For this review, take the finished solid that the model builds, in its own axes (mm). A direction names the side the tool comes from. Coordinates: 2 decimals unless noted, no trailing zeros. Loops run counter-clockwise (first coordinate to the right, second up) from the corner with the lowest first, then second, coordinate; pieces in that order, holes last.
1. Take a section at B-B, the plane y = -2. State the section outline as (x, z) points, then the cut area to 3 significant figures.
2. To check wall thickness, follow probe 1 along Y at (x, z) = (0, 42); probe 2 along Z at (x, y) = (10, 0); probe 3 along Y at (x, z) = (-9, 43.5). State the ranges of each line that lie inside material, in increasing order.
3. Clearance check with flat-ended pins moving along their axes: P1, Ø2.5, axis at y = -9.5, z = 8, coming from the +X side; P2, Ø8, axis at x = -5, z = 22, coming from the +Y side; P3, Ø8, axis at y = 5, z = 23, coming from the +X side; P4, Ø4, axis at x = 6, y = 24.5, coming from the -Z side. State where each tip first meets the part, or that it passes through.
4. Take a section at A-A, the plane x = -3.5. State the section outline as (y, z) points.
5. Take a section at D-D, the plane y = 23.5. State the section outline as (x, z) points, then the cut area to 3 significant figures.
6. Mouldability with a two-part tool opening along Y and no side actions: class faces 1 (the face through (-10.319, -9, 25)), 2 (the face through (0, -11, 6.35)), 3 (the face through (9, -10.319, 25)) as pulls with the +Y half, pulls with the -Y half, needs draft (parallel to the pull), parting line crosses it, or undercut.
7. Machinability: for faces 4 (the face through (0.593, 24.74, 3.188)), 5 (the face through (-9.79, 8.96, 7.67)), 6 (the face through (-0.1, -12.7, 10.4)), which of the approach directions +Z, -Z, +X, -X, +Y, -Y give a long, thin tool a straight path to every point of the face, cutting with its end or side? Answer none if there is none.
8. Take a section at C-C, the plane z = 35. State the section outline as (x, y) points.
```python
from build123d import *

# Parameters (mm, degrees)
SKETCH1_R               = 16.66875
BOSS_EXTRUDE1_DEPTH     = 50.8
SKETCH2_R               = 16.66875
BOSS_EXTRUDE2_DEPTH     = 34.13125
SKETCH3_R               = 16.66875
BOSS_EXTRUDE3_DEPTH     = 34.13125
CUT_EXTRUDE1_DEPTH      = 71.075134343
CUT_EXTRUDE1_DEPTH_BACK = 71.075134343
CUT_EXTRUDE2_DEPTH      = 80.537552304
SKETCH8_R               = 12.7
CUT_EXTRUDE3_DEPTH      = 44.45
SKETCH9_R               = 13.49375
CUT_EXTRUDE4_DEPTH      = 19.05
SKETCH10_R              = 12.7
CUT_EXTRUDE5_DEPTH      = 44.45
SKETCH11_R              = 13.49375
CUT_EXTRUDE6_DEPTH      = 19.05
SKETCH12_R              = 12.7
CUT_EXTRUDE7_DEPTH      = 44.45
SKETCH13_R              = 13.49375
CUT_EXTRUDE8_DEPTH      = 19.05


with BuildPart() as part:
    # Sketch1 → Boss-Extrude1 (new body)
    with BuildSketch(Plane.XY):
        Circle(SKETCH1_R)
    extrude(amount=BOSS_EXTRUDE1_DEPTH)

    # Sketch2 → Boss-Extrude2 (add)
    with BuildSketch(Plane(origin=(0, 0, 0), x_dir=(0, 0, -1), z_dir=(1, 0, 0))):
        with Locations((-16.66875, 0)):
            Circle(SKETCH2_R)
    extrude(amount=BOSS_EXTRUDE2_DEPTH)

    # Sketch3 → Boss-Extrude3 (add)
    with BuildSketch(Plane(origin=(0, 0, 0), x_dir=(1, 0, 0), z_dir=(0, 1, 0))):
        with Locations(Location((0, -16.66875, 0), (0, 0, 90))):
            Circle(SKETCH3_R)
    extrude(amount=BOSS_EXTRUDE3_DEPTH)

    # Sketch4 → Cut-Extrude1 (cut, two sides: drawn at the far end of the back side and taken through both)
    with BuildSketch(Plane(origin=(0, 0, 0), x_dir=(1, 0, 0), z_dir=(0, 1, 0)).offset(-CUT_EXTRUDE1_DEPTH_BACK)):
        with BuildLine():
            Line((-16.66875, -16.66875), (-16.66875, 0))
            Line((-16.66875, 0), (0, 0))
            ThreePointArc((0, 0), (-11.786586159, -4.882163841), (-16.66875, -16.66875))
        make_face()
    extrude(amount=CUT_EXTRUDE1_DEPTH + CUT_EXTRUDE1_DEPTH_BACK, mode=Mode.SUBTRACT)

    # Sketch5 → Cut-Extrude2 (cut, through all)
    with BuildSketch(Plane(origin=(34.13125, 0, 0), x_dir=(0, 0, -1), z_dir=(1, 0, 0))):
        with BuildLine():
            Line((-16.66875, -16.66875), (0, -16.66875))
            Line((0, -16.66875), (0, 0))
            ThreePointArc((0, 0), (-4.882163841, -11.786586159), (-16.66875, -16.66875))
        make_face()
    extrude(amount=-CUT_EXTRUDE2_DEPTH, mode=Mode.SUBTRACT)

    # Sketch8 → Cut-Extrude3 (cut)
    with BuildSketch(Plane(origin=(0, 34.13125, 0), x_dir=(1, 0, 0), z_dir=(0, 1, 0))):
        with Locations(Location((0, -16.66875, 0), (0, 0, 270))):
            Circle(SKETCH8_R)
    extrude(amount=-CUT_EXTRUDE3_DEPTH, mode=Mode.SUBTRACT)

    # Sketch9 → Cut-Extrude4 (cut)
    with BuildSketch(Plane(origin=(0, 34.13125, 0), x_dir=(1, 0, 0), z_dir=(0, 1, 0))):
        with Locations(Location((0, -16.66875, 0), (0, 0, 270))):
            Circle(SKETCH9_R)
    extrude(amount=-CUT_EXTRUDE4_DEPTH, mode=Mode.SUBTRACT)

    # Sketch10 → Cut-Extrude5 (cut)
    with BuildSketch(Plane(origin=(34.13125, 0, 0), x_dir=(0, 0, -1), z_dir=(1, 0, 0))):
        with Locations((-16.66875, 0)):
            Circle(SKETCH10_R)
    extrude(amount=-CUT_EXTRUDE5_DEPTH, mode=Mode.SUBTRACT)

    # Sketch11 → Cut-Extrude6 (cut)
    with BuildSketch(Plane(origin=(34.13125, 0, 0), x_dir=(0, 0, -1), z_dir=(1, 0, 0))):
        with Locations((-16.66875, 0)):
            Circle(SKETCH11_R)
    extrude(amount=-CUT_EXTRUDE6_DEPTH, mode=Mode.SUBTRACT)

    # Sketch12 → Cut-Extrude7 (cut)
    with BuildSketch(Plane.XY.offset(50.8)):
        Circle(SKETCH12_R)
    extrude(amount=-CUT_EXTRUDE7_DEPTH, mode=Mode.SUBTRACT)

    # Sketch13 → Cut-Extrude8 (cut)
    with BuildSketch(Plane.XY.offset(50.8)):
        Circle(SKETCH13_R)
    extrude(amount=-CUT_EXTRUDE8_DEPTH, mode=Mode.SUBTRACT)


solid = part.part
```
Results list:
1. outline: (-16.55, 14.67) arc R16.67 ccw to (-2, 0.12) - (34.13, 0.12) - (34.13, 3.32) - (15.08, 3.32) - (15.08, 4.13) - (2, 4.13) arc R12.7 cw to (-2, 4.13) - (-10.32, 4.13) - (-10.32, 6.35) - (-12.54, 6.35) - (-12.54, 14.67) arc R12.7 cw to (-12.54, 18.67) - (-12.54, 31.75) - (-13.34, 31.75) - (-13.34, 50.8) - (-16.55, 50.8) - close; (12.54, 29.21) - (15.08, 29.21) - (15.08, 30.01) - (34.13, 30.01) - (34.13, 33.22) - (16.55, 33.22) - (16.55, 50.8) - (13.34, 50.8) - (13.34, 31.75) - (12.54, 31.75) - close
1. area: 434 mm2
2. probe 1: y = -16.67 to -13.49, 13.49 to 16.67
2. probe 2: z = 0 to 3.97
2. probe 3: y = -14.03 to -10.05, 10.05 to 14.03
3. P1: stops at x = 34.13
3. P2: stops at y = -10.32
3. P3: stops at x = -10.32
3. P4: stops at z = 0.49
4. outline: (-16.3, 13.17) arc R16.67 ccw to (-3.5, 0.37) - (34.13, 0.37) - (34.13, 3.64) - (15.08, 3.64) - (15.08, 4.46) - (3.5, 4.46) arc R12.7 cw to (-3.5, 4.46) - (-10.32, 4.46) - (-10.32, 6.35) - (-12.21, 6.35) - (-12.21, 13.17) arc R12.7 cw to (-12.21, 20.17) - (-12.21, 31.75) - (-13.03, 31.75) - (-13.03, 50.8) - (-16.3, 50.8) - close; (12.21, 28.88) - (15.08, 28.88) - (15.08, 29.7) - (34.13, 29.7) - (34.13, 32.97) - (16.3, 32.97) - (16.3, 50.8) - (13.03, 50.8) - (13.03, 31.75) - (12.21, 31.75) - close
5. outline: circle Ø33.34 at (0, 16.67); hole circle Ø26.99 at (0, 16.67)
5. area: 301 mm2
6. face 1: undercut
6. face 2: needs draft
6. face 3: pulls with the +Y half
7. face 4: +Y
7. face 5: +X
7. face 6: +Z, +Y
8. outline: circle Ø33.34 at (0, 0); hole circle Ø26.99 at (0, 0)
